The figure shows three views and two pictorial views of one solid part (mm, origin at its lowest corner). Answer the questions. A direction names the side the tool comes from. Coordinates: 2 decimals unless noted, no trailing zeros. Loops run counter-clockwise (first coordinate to the right, second up) from the corner with the lowest first, then second, coordinate; pieces in that order, holes last. Notation, with made-up numbers: M 82,10.25 L 90,10.25 A26 cw 90,38.25 Z; hole C -8,7 d5. An arc over 180 degrees is marked long. Answer as a JSON object with one key per item and string values. Group by question number.
1. A straight line is drawn through the part: L1, parallel to Z at x = 24.5, y = 98. Find the intervals that lie inside material, in ascending order.
2. Given pin 1 (19 mm diameter, centred on x = 42.5, y = 57.5, fed in from +Z); pin 2 (3 mm diameter, centred on x = 24.5, z = 104, fed in from -Y), each flat-ended and moving along its own axis, determine where each tip first touches the part or whether it passes through.
3. For the marked faces 1 and 2, determine the directions among +Z, -Z, +X, -X, +Y, -Y from which every point of the face is accessible in a straight line to the end or side of a thin tool.
4. A cutting plane is placed at B-B on y = 61. Give the vertices of the cut face in (x, z).
5. A cutting plane is placed at A-A on x = 47. Give the vertices of the cut face in (y, z), and give its area (3 significant figures).
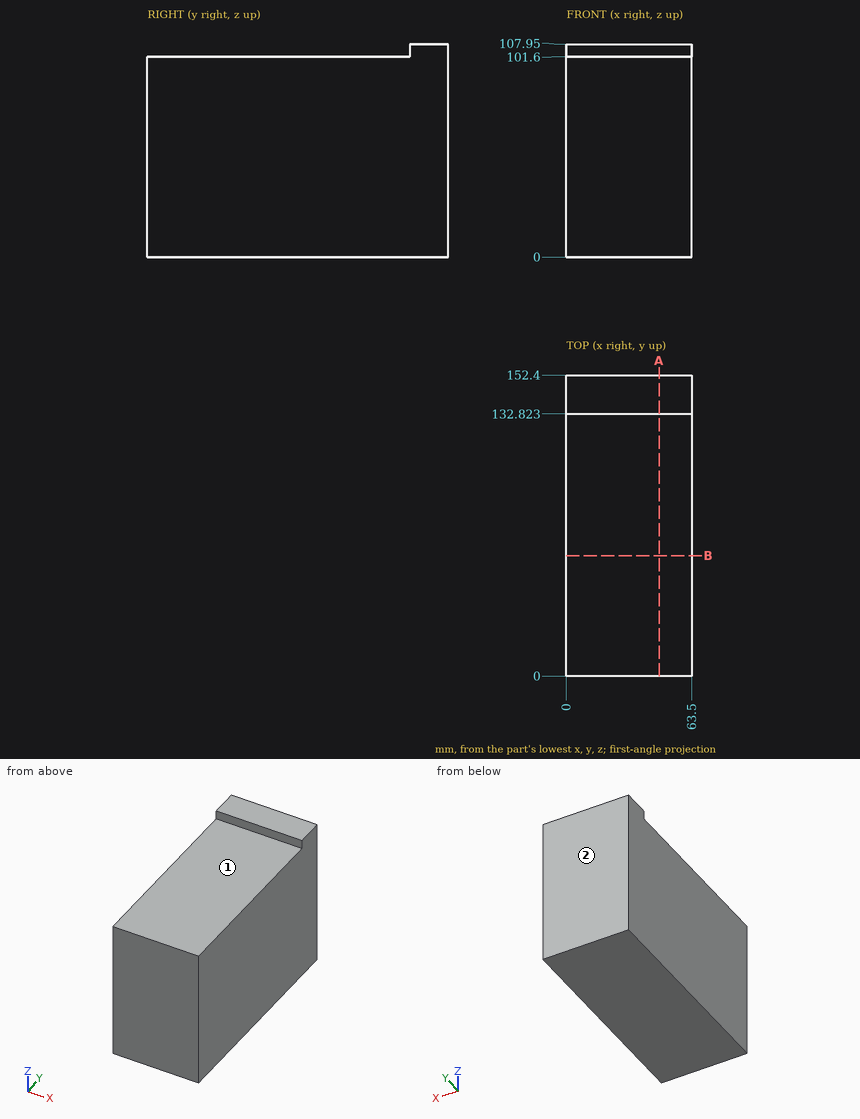
From the geometry:
{
 "1": {"L1": "z = 0 to 101.6"},
 "2": {"pin 1": "stops at z = 101.6", "pin 2": "stops at y = 132.82"},
 "3": {"face 1": "+Z, +X, -X, -Y", "face 2": "+Z, -Z, +X, -X, +Y"},
 "4": {"outline": "M 0,0 L 63.5,0 L 63.5,101.6 L 0,101.6 Z"},
 "5": {"outline": "M 0,0 L 152.4,0 L 152.4,107.95 L 132.82,107.95 L 132.82,101.6 L 0,101.6 Z", "area": "15,600 mm²"}
}
